Build history of the part. All positions in model axes, mm. A direction names the side the tool comes from. Give positions to 0.01 mm unless a question says otherwise; leave off trailing zeros. Loops run counter-clockwise (first coordinate to the right, second up) from the corner with the lowest first, then second, coordinate; pieces in that order, holes last. Notation, with made-up numbers: M -4,49.25 L 12,49.25 A25 cw 12,61.25 Z; hole C 82.25,-4.5 d5. An arc over 180 degrees is marked long. Put each result on its own line as item: value.
```python
from build123d import *

# Parameters (mm, degrees)
EXTRUDE_1_DEPTH     = 4
SKETCH_3_R          = 7
EXTRUDE_2_DEPTH     = 21.2
SKETCH_4_R          = 5.851481146
EXTRUDE_3_DEPTH     = 2.2
SKETCH_5_R          = 6.392993162
EXTRUDE_4_DEPTH     = 0.8
SKETCH_6_R          = 3
CUT_EXTRUDE_1_DEPTH = 58.8


with BuildPart() as part:
    # 草图1 → 旋转1 (revolve)
    with BuildSketch(Plane.XY, mode=Mode.PRIVATE) as revolve_1_sk:
        with BuildLine():
            Line((0, -11.727997448), (-8.526388877, -11.727997448))
            Line((-8.526388877, -11.727997448), (-11.247580715, -15.435038577))
            Line((-11.247580715, -15.435038577), (-11.247580715, -21.146383116))
            add(Edge.make_bspline(
                [(-11.247580715, -21.146383116), (-9.369073773, -21.8008603), (-10.889689746, -25.079347996), (-18.519348405, -26.382423308), (-13.657626369, -29.045080289), (-17.728346259, -31.072774498), (-17.5, -32.027997448)],
                knots=[0, 0, 0, 0, 0.239282786, 0.633272554, 0.728833694, 1, 1, 1, 1], degree=3))
            Line((-17.5, -32.027997448), (-16.297611676, -32.027997448))
            Line((-16.297611676, -32.027997448), (-8.268926003, -26.138136704))
            Line((-8.268926003, -26.138136704), (-8.268926003, -20.454901012))
            Line((-8.268926003, -20.454901012), (-10.045192391, -19.845982903))
            Line((-10.045192391, -19.845982903), (-10.045192391, -16.111285163))
            Line((-10.045192391, -16.111285163), (-8.268926003, -13.47264002))
            Line((-8.268926003, -13.47264002), (0, -13.47264002))
            Line((0, -13.47264002), (0, -11.727997448))
        make_face()
    revolve(revolve_1_sk.sketch.rotate(Axis((0, 56.825270067, 0), (0, -1, 0)), 270), axis=Axis((0, 56.825270067, 0), (0, -1, 0)))

    # 草图2 → 凸台-拉伸1 (add)
    with BuildSketch(Plane(origin=(0, -11.727997448, 0), x_dir=(1, 0, 0), z_dir=(0, 1, 0))):
        Polygon((4.810541209, 6.495538978), (-3.220031161, 7.413820382), (-8.03057237, 0.918281404), (-4.810541209, -6.495538978), (3.220031161, -7.413820382), (8.03057237, -0.918281404), align=None)
    extrude(amount=EXTRUDE_1_DEPTH)

    # 草图3 → 凸台-拉伸2 (add)
    with BuildSketch(Plane(origin=(0, -7.727997448, 0), x_dir=(1, 0, 0), z_dir=(0, 1, 0))):
        with Locations(Location((0, 0, 0), (0, 0, 83.476664908))):
            Circle(SKETCH_3_R)
    extrude(amount=EXTRUDE_2_DEPTH)

    # 草图4 → 凸台-拉伸3 (add)
    with BuildSketch(Plane(origin=(0, 13.472002552, 0), x_dir=(1, 0, 0), z_dir=(0, 1, 0))):
        with Locations(Location((0, 0, 0), (0, 0, 270))):
            Circle(SKETCH_4_R)
    extrude(amount=EXTRUDE_3_DEPTH)

    # 草图5 → 凸台-拉伸4 (add)
    with BuildSketch(Plane(origin=(0, 15.672002552, 0), x_dir=(1, 0, 0), z_dir=(0, 1, 0))):
        with Locations(Location((0, 0, 0), (0, 0, 270))):
            Circle(SKETCH_5_R)
    extrude(amount=EXTRUDE_4_DEPTH)

    # 草图6 → 切除-拉伸1 (cut)
    with BuildSketch(Plane(origin=(0, 16.472002552, 0), x_dir=(1, 0, 0), z_dir=(0, 1, 0))):
        with Locations(Location((0, 0, 0), (0, 0, 270))):
            Circle(SKETCH_6_R)
    extrude(amount=-CUT_EXTRUDE_1_DEPTH, mode=Mode.SUBTRACT)


solid = part.part
```
Q1. Slice it at A-A (y = -10). List the corners of the cut face in (x, z).
Here are the results:
outline: M -8.03,-0.92 L -3.22,-7.41 L 4.81,-6.5 L 8.03,0.92 L 3.22,7.41 L -4.81,6.5 Z; hole C 0,0 d6
Q2. Drop flat-ended pins along their axis: pin 1 Ø5 at (x, y) = (-5, -14.5) entering from -Z; pin 2 Ø3.5 at (x, z) = (-2.5, -6) entering from +Y; pin 3 Ø12 at (y, z) = (-22, 13.5) entering from +X; pin 4 Ø1.5 at (x, z) = (12, -3) entering from +Y. Give the stop position or say it passes through.
Here are the results:
pin 1: z = -10.92
pin 2: y = 16.47
pin 3: x = 13.18
pin 4: y = -24.22
Q3. Probe line 1 (X direction, y = 2, z = 0); line 2 (Y direction, x = 3, z = 3.5); line 3 (Y direction, x = -9, z = -5.5). List the from-to ranges inside material, lowest first. Write a range as from..to.
Here are the results:
line 1: -7..-3, 3..7
line 2: -13.47..16.47
line 3: -27.81..-23.36, -21.49..-14.48
Q4. Slice it at B-B (y = -5). List the corners of the cut face in (x, z).
Here are the results:
outline: C 0,0 d14; hole C 0,0 d6
Q5. Mould opens along X. For faces 5 (the cylindrical face through (-5.19, 14.56, 2.7)), 6 (the flat face through (6.44, -9.76, -2.74)), 7 (the conical face through (-8.284, -13.601, -1.088)), 8 (the flat face through (-4, -7.728, 6)) say: pulls with the +X half, pulls with the -X half, needs draft (parallel to the pull), parting line crosses it, or undercut.
Here are the results:
face 5: parting line crosses it
face 6: pulls with the +X half
face 7: undercut
face 8: needs draft
Q6. Tool access for faces 1 (the flat face through (-1.9, 15.672, 5.7)), 2 (the flat face through (-2, -11.728, 7)), 3 (the flat face through (5.6, -9.8, 4.2)), 4 (the flat face through (4, -7.728, -6)): list every direction of +Z, -Z, +X, -X, +Y, -Y with a clear straight run to the whole face (end or side of a thin tool).
Here are the results:
face 1: none
face 2: +Y
face 3: +Z, +X, +Y
face 4: -Z, +X, +Y
